Could you check a few things on this drawing? It's one solid part, dimensions in mm from its lowest x, y, z. Give positions to 0.01 mm unless a question says otherwise; leave off trailing zeros. Loops run counter-clockwise (first coordinate to the right, second up) from the corner with the lowest first, then second, coordinate; pieces in that order, holes last. Notation, with made-up numbers: (48, 8.25) -> (62, 8.25) arc R29 cw to (62, 31.25) -> close; hole circle Ø6 at (-14.75, 58.25). An arc over 180 degrees is marked (long way). Use CSV: the item, a comma, the result in double quotes.
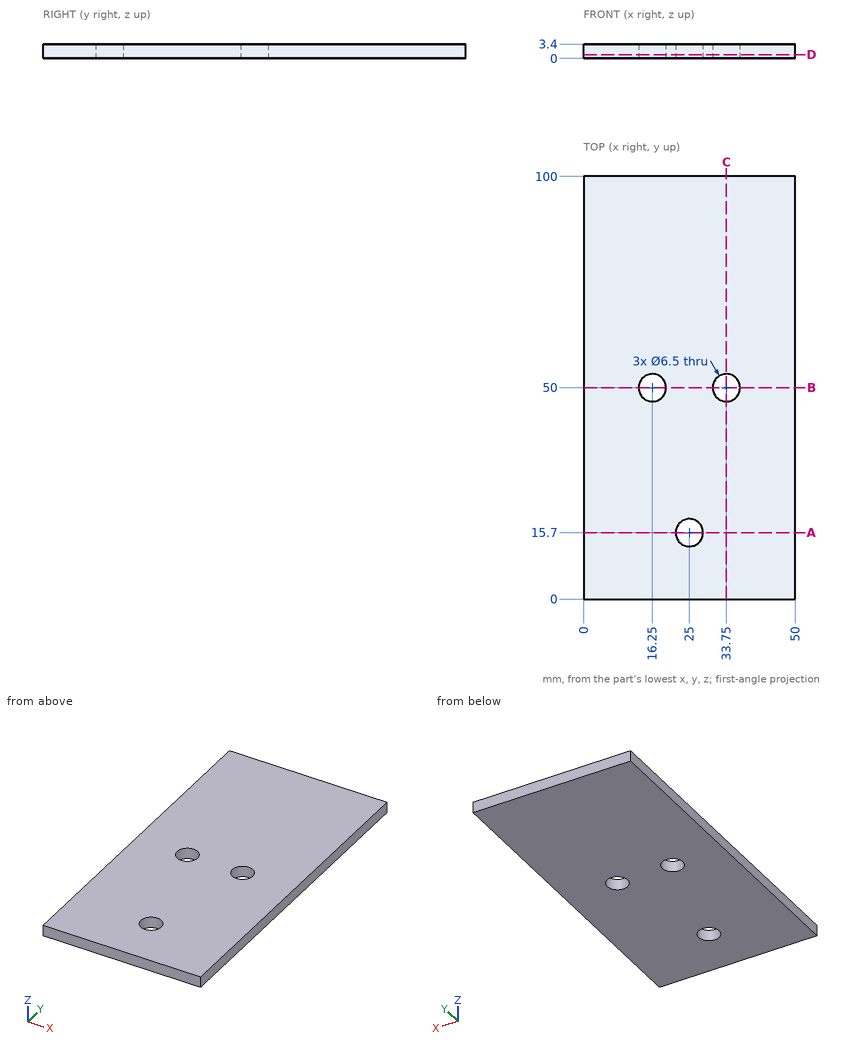
(1) If we section it at C-C, the plane x = 33.75: Write out the boundary of the cut face in (y, z).
Answer sheet:
outline,"(0, 0) -> (46.75, 0) -> (46.75, 3.4) -> (0, 3.4) -> close; (53.25, 0) -> (100, 0) -> (100, 3.4) -> (53.25, 3.4) -> close"
(2) If we section it at D-D, the plane z = 0.9: Write out the boundary of the cut face in (x, y).
Answer sheet:
outline,"(0, 0) -> (50, 0) -> (50, 100) -> (0, 100) -> close; hole circle Ø6.5 at (16.25, 50); hole circle Ø6.5 at (25, 15.7); hole circle Ø6.5 at (33.75, 50)"
(3) If I drill on L1, parallel to Y at x = 25, z = 1.6; L2, parallel to Y at x = 33.75, z = 1.55, over which ranges is the centre line in solid material (lowest first)? Write a range as from..to.
Answer sheet:
L1,"y = 0..12.45, 18.95..100"
L2,"y = 0..46.75, 53.25..100"
(4) If we section it at A-A, the plane y = 15.7: Write out the boundary of the cut face in (x, z).
Answer sheet:
outline,"(0, 0) -> (21.75, 0) -> (21.75, 3.4) -> (0, 3.4) -> close; (28.25, 0) -> (50, 0) -> (50, 3.4) -> (28.25, 3.4) -> close"
(5) If we section it at B-B, the plane y = 50: Write out the boundary of the cut face in (x, z).
Answer sheet:
outline,"(0, 0) -> (13, 0) -> (13, 3.4) -> (0, 3.4) -> close; (19.5, 0) -> (30.5, 0) -> (30.5, 3.4) -> (19.5, 3.4) -> close; (37, 0) -> (50, 0) -> (50, 3.4) -> (37, 3.4) -> close"
